Input: part model. Units: mm. Frame: model coordinates. Round coordinates to 2 decimals unless told otherwise and drop trailing zeros. Use a Markdown table: item, result.
Autodesk Inventor part; units mm, degrees
ref_plane "C1_XY" through (0, 0, 0) normal (0, 0, 1) x (1, 0, 0)
ref_plane "C1_YZ" through (0, 0, 0) normal (1, 0, 0) x (0, 1, 0)
ref_plane "C1_ZX" through (0, 0, 0) normal (0, 1, 0) x (0, 0, 1)
sketch "Sketch_1" plane through (0, 0, 0) normal (0, 0, 1) x (1, 0, 0)
  line L0 (-10, -7) -> (-8, -7)
  line L1 (-8, -7) -> (-8, -4)
  line L2 (-8, -4) -> (-7.0607, -4)
  line L3 (-7.0607, -4) -> (-4, -7.0607)
  line L4 (-4, -7.0607) -> (-4, -9.4804)
  line L5 (-4, -9.4804) -> (-3.7, -10)
  line L6 (-3.7, -10) -> (-4, -10.5196)
  line L7 (-4, -10.5196) -> (-4, -12.9393)
  line L8 (-4, -12.9393) -> (-7.0607, -16)
  line L9 (-7.0607, -16) -> (-8, -16)
  line L10 (-8, -16) -> (-8, -13)
  line L11 (-8, -13) -> (-10, -13)
  line L12 (-10, -13) -> (-10, -19)
  arc A0 (-10, -19) -> (-9, -20) centre (-9, -19) ccw
  line L13 (-9, -20) -> (-3, -20)
  line L14 (-3, -20) -> (-3, -18)
  line L15 (-3, -18) -> (-6, -18)
  line L16 (-6, -18) -> (-6, -17.0607)
  line L17 (-6, -17.0607) -> (-2.9393, -14)
  line L18 (-2.9393, -14) -> (-0.5196, -14)
  line L19 (-0.5196, -14) -> (0, -13.7)
  line L20 (0, -13.7) -> (0.5196, -14)
  line L21 (0.5196, -14) -> (2.9393, -14)
  line L22 (2.9393, -14) -> (6, -17.0607)
  line L23 (6, -17.0607) -> (6, -18)
  line L24 (6, -18) -> (3, -18)
  line L25 (3, -18) -> (3, -20)
  line L26 (3, -20) -> (9, -20)
  arc A1 (9, -20) -> (10, -19) centre (9, -19) ccw
  line L27 (10, -19) -> (10, -13)
  line L28 (10, -13) -> (8, -13)
  line L29 (8, -13) -> (8, -16)
  line L30 (8, -16) -> (7.0607, -16)
  line L31 (7.0607, -16) -> (4, -12.9393)
  line L32 (4, -12.9393) -> (4, -10.5196)
  line L33 (4, -10.5196) -> (3.7, -10)
  line L34 (3.7, -10) -> (4, -9.4804)
  line L35 (4, -9.4804) -> (4, -7.0607)
  line L36 (4, -7.0607) -> (7.0607, -4)
  line L37 (7.0607, -4) -> (8, -4)
  line L38 (8, -4) -> (8, -7)
  line L39 (8, -7) -> (10, -7)
  line L40 (10, -7) -> (10, 7)
  line L41 (10, 7) -> (8, 7)
  line L42 (8, 7) -> (8, 4)
  line L43 (8, 4) -> (7.0607, 4)
  line L44 (7.0607, 4) -> (4, 7.0607)
  line L45 (4, 7.0607) -> (4, 9.4804)
  line L46 (4, 9.4804) -> (3.7, 10)
  line L47 (3.7, 10) -> (4, 10.5196)
  line L48 (4, 10.5196) -> (4, 12.9393)
  line L49 (4, 12.9393) -> (7.0607, 16)
  line L50 (7.0607, 16) -> (8, 16)
  line L51 (8, 16) -> (8, 13)
  line L52 (8, 13) -> (10, 13)
  line L53 (10, 13) -> (10, 19)
  arc A2 (10, 19) -> (9, 20) centre (9, 19) ccw
  line L54 (9, 20) -> (3, 20)
  line L55 (3, 20) -> (3, 18)
  line L56 (3, 18) -> (6, 18)
  line L57 (6, 18) -> (6, 17.0607)
  line L58 (6, 17.0607) -> (2.9393, 14)
  line L59 (2.9393, 14) -> (0.5196, 14)
  line L60 (0.5196, 14) -> (0, 13.7)
  line L61 (0, 13.7) -> (-0.5196, 14)
  line L62 (-0.5196, 14) -> (-2.9393, 14)
  line L63 (-2.9393, 14) -> (-6, 17.0607)
  line L64 (-6, 17.0607) -> (-6, 18)
  line L65 (-6, 18) -> (-3, 18)
  line L66 (-3, 18) -> (-3, 20)
  line L67 (-3, 20) -> (-9, 20)
  arc A3 (-9, 20) -> (-10, 19) centre (-9, 19) ccw
  line L68 (-10, 19) -> (-10, 13)
  line L69 (-10, 13) -> (-8, 13)
  line L70 (-8, 13) -> (-8, 16)
  line L71 (-8, 16) -> (-7.0607, 16)
  line L72 (-7.0607, 16) -> (-4, 12.9393)
  line L73 (-4, 12.9393) -> (-4, 10.5196)
  line L74 (-4, 10.5196) -> (-3.7, 10)
  line L75 (-3.7, 10) -> (-4, 9.4804)
  line L76 (-4, 9.4804) -> (-4, 7.0607)
  line L77 (-4, 7.0607) -> (-7.0607, 4)
  line L78 (-7.0607, 4) -> (-8, 4)
  line L79 (-8, 4) -> (-8, 7)
  line L80 (-8, 7) -> (-10, 7)
  line L81 (-10, 7) -> (-10, -7)
  line L82 (-8, 1.7) -> (-8, -1.7)
  arc A4 (-8, -1.7) -> (-7.7, -2) centre (-7.7, -1.7) ccw
  line L83 (-7.7, -2) -> (-7.0636, -2)
  arc A5 (-6.8515, -2.0879) -> (-7.0636, -2) centre (-7.0636, -2.3) ccw
  line L84 (-6.8515, -2.0879) -> (-2.9393, -6)
  line L85 (-2.9393, -6) -> (2.9393, -6)
  line L86 (2.9393, -6) -> (6.8515, -2.0879)
  arc A6 (7.0636, -2) -> (6.8515, -2.0879) centre (7.0636, -2.3) ccw
  line L87 (7.0636, -2) -> (7.7, -2)
  arc A7 (7.7, -2) -> (8, -1.7) centre (7.7, -1.7) ccw
  line L88 (8, -1.7) -> (8, 1.7)
  arc A8 (8, 1.7) -> (7.7, 2) centre (7.7, 1.7) ccw
  line L89 (7.7, 2) -> (7.0636, 2)
  arc A9 (6.8515, 2.0879) -> (7.0636, 2) centre (7.0636, 2.3) ccw
  line L90 (6.8515, 2.0879) -> (2.9393, 6)
  line L91 (2.9393, 6) -> (-2.9393, 6)
  line L92 (-2.9393, 6) -> (-6.8515, 2.0879)
  arc A10 (-7.0636, 2) -> (-6.8515, 2.0879) centre (-7.0636, 2.3) ccw
  line L93 (-7.0636, 2) -> (-7.7, 2)
  arc A11 (-7.7, 2) -> (-8, 1.7) centre (-7.7, 1.7) ccw
extrude "Extrusion1" add sketch "Sketch_1" against normal blind 520
sketch "Sketch2" plane through (0, 0, -520) normal (0, 0, -1) x (-1, 0, 0)
  point P0 (0, 10)
hole "Hole1" at (0, 10, -520) direction (0, 0, 1) diameter 4.2 depth 520
pattern_linear "Rectangular Pattern1" count 2 spacing 20 along (0, -1, 0) of "Hole1"
ref_plane "C1_XY" through (0, 0, 0) normal (0, 0, 1) x (1, 0, 0)
ref_plane "C1_YZ" through (0, 0, 0) normal (1, 0, 0) x (0, 1, 0)
ref_plane "C1_ZX" through (0, 0, 0) normal (0, 1, 0) x (0, 0, 1)
properties part number "HFS5-2040-520"
1) Cut plane A-A on z = -331. Count the separate pieces of the cut face and the enclosed holes in it, and give its area (3 significant figures).
Results found:
| item | result |
|---|---|
| separate pieces | 1 |
| enclosed holes | 3 |
| area | 324 mm² |
2) Pin query (flat end, axial travel): pin 1 Ø1.2 at (x, z) = (1.5, -307.5) entering from +Y; pin 2 Ø0.6 at (y, z) = (-19.5, -353.5) entering from +X; pin 3 Ø1.2 at (x, z) = (2, -344.5) entering from -Y. Return the tip coordinate at first contact, or that it passes through.
Results found:
| item | result |
|---|---|
| pin 1 | stops at y = 14 |
| pin 2 | stops at x = 9.98 |
| pin 3 | stops at y = -14 |
3) Line query: L1, parallel to Y at x = 0, z = -308; L2, parallel to Y at x = -8.25, z = -257.5; L3, parallel to Y at x = -0.5, z = -123. Output: solid intervals per line, ascending. Write a range as [from, to].
Results found:
| item | result |
|---|---|
| L1 | y = [-13.7, -12.1], [-7.9, -6], [6, 7.9], [12.1, 13.7] |
| L2 | y = [-20, -13], [-7, 7], [13, 20] |
| L3 | y = [-13.99, -12.04], [-7.96, -6], [6, 7.96], [12.04, 13.99] |
